Source: CAD feature listing. Evaluate the final solid. Frame: model axes, mm. Round coordinates to 2 decimals unless told otherwise and drop trailing zeros. Loops run counter-clockwise (first coordinate to the right, second up) from the corner with the lowest first, then second, coordinate; pieces in that order, holes last.
Item 1: Section query D-D on x = -5.75. Return loops of the section in (y, z).
Item 2: Ray query, L1, parallel to Z at x = -1.25, y = 17; L2, parallel to Y at x = -7.75, z = 4; L3, parallel to Y at x = -5.5, z = -14.75. Return the intervals inside material, ascending.
Item 3: Section query C-C on x = 7.5. Return loops of the section in (y, z).
Item 4: Section query B-B on y = -5. Return loops of the section in (x, z), then the cut area to 3 significant figures.
Item 5: Section query A-A on x = 2. Return loops of the section in (y, z), then the cut area to 3 significant figures.
Item 6: Pull-direction query (Y, two-part tool) for faces 1 (the flat face through (-0.75, -9.522, -9.265)), 2 (the flat face through (-1, 6, 0)), 3 (the cylindrical face through (-4.456, 10.503, 2.465)), 4 (the cylindrical face through (-9.187, 12.084, 2.465)); classes: released by +Y, released by -Y, zero draft, split by the parting line, or undercut.
Item 7: First-contact query: P1, Ø1.5, axis at y = 21, z = 0, coming from the +X side; P2, Ø1, axis at x = -10, z = -5, coming from the +Y side; P3, Ø6, axis at x = 8.5, y = 19.5, coming from the -Z side; P4, Ø4, axis at y = 12, z = 0.5, coming from the -X side. Flat tips, straight axial feed; report the tip coordinate or a pass-through.
```python
from build123d import *

# Parameters (mm, degrees)
ESQUISSE1_R             = 1.75
ESQUISSE1_R_2           = 3.5
BOSS_EXTRU_1_DEPTH      = 5
ENL_V_MAT_EXTRU_2_REACH = 41.592
BOSS_EXTRU_2_DEPTH      = 30
ESQUISSE5_W             = 30
ESQUISSE5_H             = 5
BOSS_EXTRU_3_DEPTH      = 20


with BuildPart() as part:
    # Esquisse1 → Boss.-Extru.1 (new body)
    with BuildSketch(Plane.XY):
        with BuildLine():
            Line((-15.959557324, 10.348837209), (-15.959557324, -9.651162791))
            Line((-15.959557324, -9.651162791), (14.040442676, -9.651162791))
            Line((14.040442676, -9.651162791), (14.040442676, 10.348837209))
            ThreePointArc((14.040442676, 10.348837209), (-0.959557324, 25.348837209), (-15.959557324, 10.348837209))
        make_face()
        with Locations((-8.959557324, 10.348837209)):
            Circle(ESQUISSE1_R, mode=Mode.SUBTRACT)
        with Locations((7.040442676, 10.348837209)):
            Circle(ESQUISSE1_R, mode=Mode.SUBTRACT)
        with Locations((-0.959557324, 10.348837209)):
            Circle(ESQUISSE1_R_2, mode=Mode.SUBTRACT)
    extrude(amount=BOSS_EXTRU_1_DEPTH)

    # Esquisse2 → Enlèv. mat.-Extru.2 (cut, up to next)
    with BuildSketch(Plane.ZY.offset(15.959557324), mode=Mode.PRIVATE) as enl_v_mat_extru_2_sk1:
        Polygon((0, -9.651162791), (0, -6.1501251), (1.274273509, -9.651162791), align=None)
    enl_v_mat_extru_2_tool1 = extrude(enl_v_mat_extru_2_sk1.sketch, amount=-ENL_V_MAT_EXTRU_2_REACH, mode=Mode.PRIVATE) & part.part
    add(enl_v_mat_extru_2_tool1.solids().sort_by_distance((-15.959557, -8.48415, 0.424758))[0], mode=Mode.SUBTRACT)

    # Esquisse4 → Boss.-Extru.2 (add)
    with BuildSketch(Plane.ZY.offset(15.959557324)):
        Polygon((5, -9.651162791), (1.710100717, -10.848588204), (1.274273509, -9.651162791), align=None)
    extrude(amount=-BOSS_EXTRU_2_DEPTH)

    # Esquisse5 → Boss.-Extru.3 (add)
    with BuildSketch(Plane(origin=(0, -0.719427971, -1.976612106), x_dir=(-1, 0, 0), z_dir=(0, -0.34202014332566333, -0.9396926207859103))):
        with Locations((0.959557324, -8.279227173)):
            Rectangle(ESQUISSE5_W, ESQUISSE5_H)
    extrude(amount=BOSS_EXTRU_3_DEPTH)


solid = part.part
```
Data:
1. outline: (-17.69, -17.08) - (-12.99, -18.79) - (-6.15, 0) - (24.56, 0) - (24.56, 5) - (-9.65, 5) - close
2. L1: z = 0 to 5
2. L2: y = -10.02 to 9.08, 11.61 to 23.72
2. L3: y = -16.84 to -11.52
3. outline: (-17.69, -17.08) - (-12.99, -18.79) - (-6.15, 0) - (8.66, 0) - (8.66, 5) - (-9.65, 5) - close; (12.04, 0) - (22.74, 0) - (22.74, 5) - (12.04, 5) - close
4. outline: (-15.96, 0) - (14.04, 0) - (14.04, 5) - (-15.96, 5) - close
4. area: 150 mm2
5. outline: (-17.69, -17.08) - (-12.99, -18.79) - (-6.15, 0) - (8.48, 0) - (8.48, 5) - (-9.65, 5) - close; (12.22, 0) - (25.05, 0) - (25.05, 5) - (12.22, 5) - close
5. area: 255 mm2
6. face 1: released by +Y
6. face 2: zero draft
6. face 3: undercut
6. face 4: undercut
7. P1: stops at x = 10.31
7. P2: stops at y = -7.79
7. P3: stops at z = 0
7. P4: stops at x = -15.96
